For this review, take the finished solid that the model builds, in its own axes (mm). Face numbers are marked on the shaded views. A direction names the side the tool comes from. Round coordinates to 2 decimals unless told otherwise and drop trailing zeros. Write each loop counter-clockwise with the first axis right and the second up, starting at its lowest first coordinate (ties: lowest second). Pieces come first, ordered by that corner, then holes. Notation, with made-up numbers: (55.25, 4.5) -> (81.25, 4.5) arc R21 ccw to (81.25, 19.5) -> close; hole circle Ø11 at (89, 23.25). An arc over 180 degrees is marked (long way). Answer in a Markdown table with one row per item.
from build123d import *

# Parameters (mm, degrees)
EXTRUDE_1_DEPTH           = 3
HOLE_WIZARD_1_D           = 2.4
HOLE_WIZARD_1_DEPTH       = 5.2
HOLE_WIZARD_1_CBORE_D     = 4.3
HOLE_WIZARD_1_CBORE_DEPTH = 2.3
HOLE_WIZARD_1_TIP         = 0.721032743


with BuildPart() as part:
    # 草图1 → 凸台-拉伸1 (new body)
    with BuildSketch(Plane.XY):
        with BuildLine():
            Line((-7.5, 2.5), (7.5, 2.5))
            ThreePointArc((7.5, 2.5), (10, 0), (7.5, -2.5))
            Line((7.5, -2.5), (-7.5, -2.5))
            ThreePointArc((-7.5, -2.5), (-10, 0), (-7.5, 2.5))
        make_face()
    extrude(amount=EXTRUDE_1_DEPTH)

    # 打孔尺寸(%根据)内六角圆柱头螺钉的类型1
    with Locations(Plane.XY.offset(3)):
        with Locations((-7.5, 0), (7.5, 0)):
            CounterBoreHole(HOLE_WIZARD_1_D / 2, HOLE_WIZARD_1_CBORE_D / 2, HOLE_WIZARD_1_CBORE_DEPTH, depth=HOLE_WIZARD_1_DEPTH)
            with Locations((0, 0, -(HOLE_WIZARD_1_DEPTH + HOLE_WIZARD_1_TIP / 2))):  # 118° drill point
                Cone(0, HOLE_WIZARD_1_D / 2, HOLE_WIZARD_1_TIP, mode=Mode.SUBTRACT)


solid = part.part
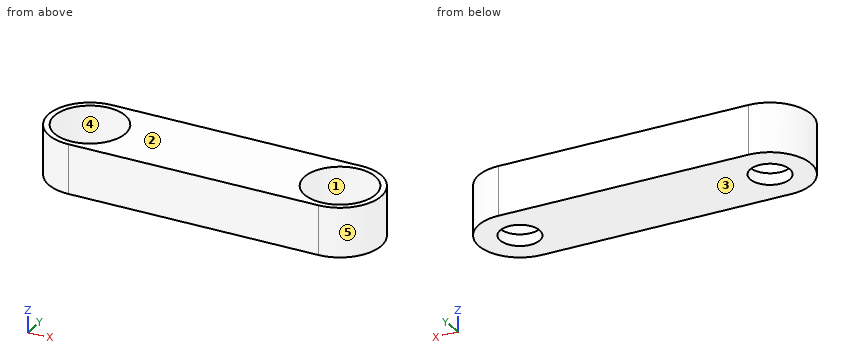
1) For the marked faces 4 and 5, list the 3-axis set-ups (+Z, -Z, +X, -X, +Y, -Y) from which the entire face can be reached by the end or side of a thin tool; tool diameter is ignored.
Solved:
| item | result |
|---|---|
| face 4 | +Z |
| face 5 | +Z, -Z, +X |
2) Consider section A-A on y = 0. State the section outline as (x, z) points.
Solved:
| item | result |
|---|---|
| outline | (-10, 0) -> (-8.7, 0) -> (-8.7, 0.7) -> (-9.65, 0.7) -> (-9.65, 3) -> (-10, 3) -> close; (-6.3, 0) -> (6.3, 0) -> (6.3, 0.7) -> (5.35, 0.7) -> (5.35, 3) -> (-5.35, 3) -> (-5.35, 0.7) -> (-6.3, 0.7) -> close; (8.7, 0) -> (10, 0) -> (10, 3) -> (9.65, 3) -> (9.65, 0.7) -> (8.7, 0.7) -> close |
3) Consider section B-B on x = -8.5. State the section outline as (y, z) points.
Solved:
| item | result |
|---|---|
| outline | (-2.29, 0) -> (-0.66, 0) -> (-0.66, 0.7) -> (-1.9, 0.7) -> (-1.9, 3) -> (-2.29, 3) -> close; (0.66, 0) -> (2.29, 0) -> (2.29, 3) -> (1.9, 3) -> (1.9, 0.7) -> (0.66, 0.7) -> close |
4) Mouldability with a two-part tool opening along Z and no side actions: class the marked faces 1, 2 and 3 as pulls with the +Z half, pulls with the -Z half, needs draft (parallel to the pull), parting line crosses it, or undercut.
Solved:
| item | result |
|---|---|
| face 1 | needs draft |
| face 2 | pulls with the +Z half |
| face 3 | pulls with the -Z half |
5) Clearance check with a flat-ended pin moving along its axis: pin 1 Ø2 at (x, y) = (-8, 1) entering from +Z. State where the tip first meets the part, or that it passes through.
Solved:
| item | result |
|---|---|
| pin 1 | z = 0.7 |
6) Consider section D-D on x = 7. State the section outline as (y, z) points.
Solved:
| item | result |
|---|---|
| outline | (-2.5, 0) -> (-1.09, 0) -> (-1.09, 0.7) -> (-2.09, 0.7) -> (-2.09, 3) -> (-2.5, 3) -> close; (1.09, 0) -> (2.5, 0) -> (2.5, 3) -> (2.09, 3) -> (2.09, 0.7) -> (1.09, 0.7) -> close |
7) For line 1 (X direction, y = -1.8, z = 2.8); line 2 (Y direction, x = -7.5, z = 0.55); line 3 (X direction, y = 1.2, z = 1.8), list the stretches that pass through material, from the lowest coordinate up. Write a range as [from, to].
Solved:
| item | result |
|---|---|
| line 1 | [-9.23, -8.68], [-6.32, 6.32], [8.68, 9.23] |
| line 2 | [-2.5, -1.2], [1.2, 2.5] |
| line 3 | [-9.69, -9.28], [-5.72, 5.72], [9.28, 9.69] |
8) Consider section C-C on z = 2.4. State the section outline as (x, y) points, then the cut area to 3 significant figures.
Solved:
| item | result |
|---|---|
| outline | (-7.5, -2.5) -> (7.5, -2.5) arc R2.5 ccw to (7.5, 2.5) -> (-7.5, 2.5) arc R2.5 ccw to start; hole circle Ø4.3 at (-7.5, 0); hole circle Ø4.3 at (7.5, 0) |
| area | 65.6 mm² |
